```python
from build123d import *

# Parameters (mm, degrees)
F0_W     = 50.8
F0_H     = 38.1
F1_DEPTH = 31.75
F3_DEPTH = 50.8
F4_W     = 25.4
F4_H     = 17.231492
F5_DEPTH = 19.05


with BuildPart() as f1:
    # F0 (on Front) → F1 (new body)
    with BuildSketch(Plane.XZ):
        with Locations((25.4, 19.05)):
            Rectangle(F0_W, F0_H)
    extrude(amount=F1_DEPTH)

    # F2 (on face) → F3 (cut)
    with BuildSketch(Plane.YZ.offset(50.8)):
        with BuildLine():
            Line((-31.75, 38.1), (-31.75, 12.7))
            ThreePointArc((-31.75, 12.7), (-16.730017, 23.080017), (-6.35, 38.1))
            Line((-6.35, 38.1), (-31.75, 38.1))
        make_face()
    extrude(amount=-F3_DEPTH, mode=Mode.SUBTRACT)

    # F4 (on face) → F5 (cut)
    with BuildSketch(Plane(origin=(0, 0, 0), x_dir=(-1, 0, 0), z_dir=(0, 1, 0))):
        with Locations((-25.4, 29.484254)):
            Rectangle(F4_W, F4_H)
    extrude(amount=-F5_DEPTH, mode=Mode.SUBTRACT)


solid = f1.part
```
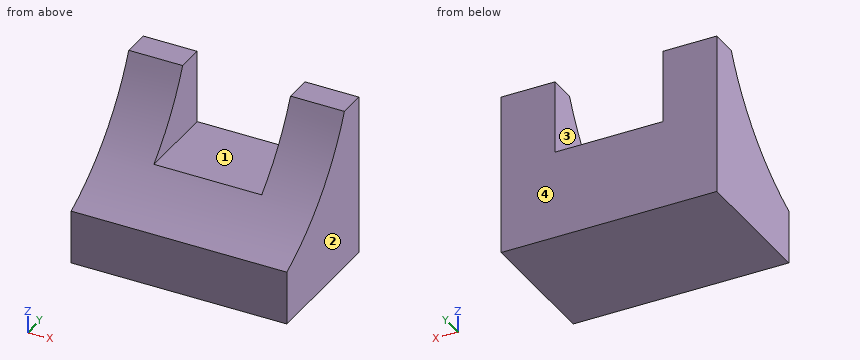
Build history of the part. All positions in model axes, mm. Face numbers are marked on the shaded views. Coordinates: 2 decimals unless noted, no trailing zeros. Write each loop counter-clockwise with the first axis right and the second up, starting at its lowest first coordinate (ties: lowest second). Pieces come first, ordered by that corner, then holes.
1. Drill centre lines: probe 1 along X at (y, z) = (-3, 22); probe 2 along Z at (x, y) = (24, -10); probe 3 along Y at (x, z) = (32, 20). Where is each one in solid material? Low to high.
Answer block:
probe 1: x = 0 to 12.7, 38.1 to 50.8
probe 2: z = 0 to 20.87
probe 3: y = -20.1 to 0
2. Band-saw the part on C-C, the plane y = -15. Give the cut face in (x, z).
Answer block:
outline: (0, 0) - (50.8, 0) - (50.8, 24.9) - (38.1, 24.9) - (38.1, 20.87) - (12.7, 20.87) - (12.7, 24.9) - (0, 24.9) - close
3. Pull direction X, two halves, no side cores. Call the marked faces 1, 2, 3 and 4: released by +X, released by -X, zero draft, split by the parting line, or undercut.
Answer block:
face 1: undercut
face 2: released by +X
face 3: undercut
face 4: zero draft
4. Drop flat-ended pins along their axis: pin 1 (15 mm diameter, centred on x = 27, y = -6.5, fed in from +Z); pin 2 (1 mm diameter, centred on x = 43, z = 28, fed in from -Y). Give the stop position or say it passes through.
Answer block:
pin 1: stops at z = 20.87
pin 2: stops at y = -12.8
5. Band-saw the part on D-D, the plane z = 34.5. Give the cut face in (x, y).
Answer block:
outline: (0, -8.15) - (12.7, -8.15) - (12.7, 0) - (0, 0) - close; (38.1, -8.15) - (50.8, -8.15) - (50.8, 0) - (38.1, 0) - close
6. Band-saw the part on A-A, the plane z = 25. Give the cut face in (x, y).
Answer block:
outline: (0, -14.91) - (12.7, -14.91) - (12.7, 0) - (0, 0) - close; (38.1, -14.91) - (50.8, -14.91) - (50.8, 0) - (38.1, 0) - close
